```python
from build123d import *

# Parameters (mm, degrees)
SKETCH1_W                = 35.980750028
SKETCH1_H                = 26
BOSS_EXTRUDE1_DEPTH      = 2
LPATTERN1_COUNT          = 2
LPATTERN1_PITCH          = 4
BOSS_EXTRUDE2_DEPTH      = 6
BOSS_EXTRUDE2_DEPTH_BACK = 12
SKETCH2_W                = 35.980750028
SKETCH2_H                = 2
FILLET1_R                = 2
FILLET2_R                = 10
SKETCH4_R                = 5
CUT_EXTRUDE1_DEPTH       = 6


with BuildPart() as part:
    # Sketch1 → Boss-Extrude1 (new body)
    with BuildSketch(Plane.XY):
        with Locations((17.990375014, 13)):
            Rectangle(SKETCH1_W, SKETCH1_H)
    extrude(amount=BOSS_EXTRUDE1_DEPTH)


with BuildPart() as lpattern1_1:
    # LPattern1: pattern copy
    add(part.part.moved(Location(Vector(0, 0, 1) * (1 * LPATTERN1_PITCH))))


with BuildPart() as part_1:
    add(part.part)

    add(lpattern1_1.part)  # Boss-Extrude2 merges LPattern1_1
    # Sketch2 → Boss-Extrude2 (add, two sides: drawn at the far end of the back side and taken through both)
    with BuildSketch(Plane(origin=(0, 0, 0), x_dir=(-1, 0, 0), z_dir=(0, 0, -1)).offset(-BOSS_EXTRUDE2_DEPTH_BACK)):
        with Locations((-17.990375014, 1)):
            Rectangle(SKETCH2_W, SKETCH2_H)
    extrude(amount=BOSS_EXTRUDE2_DEPTH + BOSS_EXTRUDE2_DEPTH_BACK)

    # Fillet1
    fillet1_edges = [part_1.edges().sort_by_distance(p)[0] for p in [
        (17.990375014, 2, 0),
        (17.990375014, 2, 6),
    ]]
    fillet(fillet1_edges, radius=FILLET1_R)

    # Fillet2
    fillet2_edges = [part_1.edges().sort_by_distance(p)[0] for p in [
        (0, 26, 5),
        (35.980750028, 26, 5),
        (0, 26, 1),
        (35.980750028, 26, 1),
    ]]
    fillet(fillet2_edges, radius=FILLET2_R)

    # Sketch4 → Cut-Extrude1 (cut)
    with BuildSketch(Plane.XY.offset(6)):
        with Locations((17.990375014, 16.77)):
            Circle(SKETCH4_R)
    extrude(amount=-CUT_EXTRUDE1_DEPTH, mode=Mode.SUBTRACT)


solid = part_1.part
```
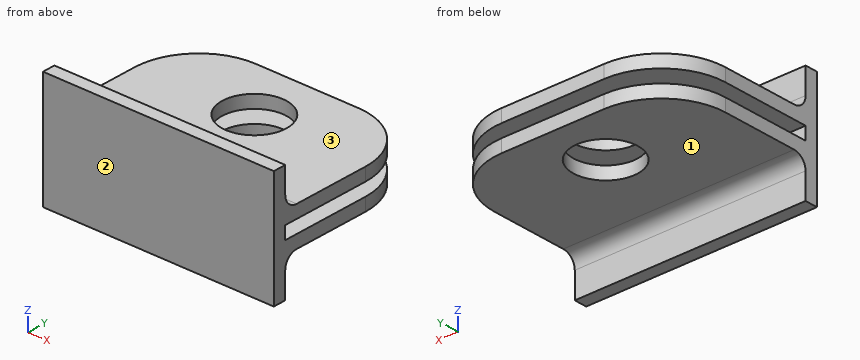
Verification items for the finished model (mm, model axes). Face numbers are marked on the shaded views. A direction names the side the tool comes from. Round coordinates to 2 decimals unless told otherwise and drop trailing zeros. Write each loop counter-clockwise with the first axis right and the second up, starting at its lowest first coordinate (ties: lowest second). Pieces come first, ordered by that corner, then holes. Notation, with made-up numbers: (11.25, 68.25) -> (56.25, 68.25) arc R26 ccw to (56.25, 95.25) -> close; hole circle Ø5 at (52.5, 24). An arc over 180 degrees is marked (long way). Write each question's results on one line, items separated by ' | '. Start each with the question number.
1. Set-up check for the marked faces 1, 2 and 3: record each of +Z, -Z, +X, -X, +Y, -Y from which the full face is reachable in a straight line by a thin tool's end or side.
2. Cross-section at B-B (x = 18). Enter the section's corners in (y, z).
3. Cross-section at D-D (x = 24.5). Enter the section's corners in (y, z).
4. Material ranges on probe 1 along Z at (x, y) = (23, 20.25); probe 2 along Y at (x, z) = (2, 3.75); probe 3 along Y at (x, z) = (22.5, 0.5), recorded low to high. Write a range as from..to.
5. Cross-section at A-A (y = 6.5). Enter the section's corners in (x, z).
6. Cross-section at C-C (y = 16.77). Enter the section's corners in (x, z).
7. Depth check by flat-ended pin: P1, Ø4.5, axis at x = 22, z = -5, coming from the +Y side; P2, Ø2, axis at x = 23.5, y = 5, coming from the -Z side; P3, Ø12, axis at x = 15.5, y = 9, coming from the +Z side; P4, Ø3, axis at x = 22.5, z = 8.5, coming from the -Y side. Enter the tip coordinate at first touch or a pass-through.
Solutions:
1) face 1: -Z, +X, -X, +Y | face 2: +Z, -Z, +X, -X, -Y | face 3: +Z, +X, -X, +Y
2) outline: (0, -6) -> (2, -6) -> (2, -2) arc R2 cw to (4, 0) -> (11.77, 0) -> (11.77, 2) -> (2, 2) -> (2, 4) -> (11.77, 4) -> (11.77, 6) -> (4, 6) arc R2 cw to (2, 8) -> (2, 12) -> (0, 12) -> close; (21.77, 0) -> (26, 0) -> (26, 2) -> (21.77, 2) -> close; (21.77, 4) -> (26, 4) -> (26, 6) -> (21.77, 6) -> close
3) outline: (0, -6) -> (2, -6) -> (2, -2) arc R2 cw to (4, 0) -> (26, 0) -> (26, 2) -> (2, 2) -> (2, 4) -> (26, 4) -> (26, 6) -> (4, 6) arc R2 cw to (2, 8) -> (2, 12) -> (0, 12) -> close
4) probe 1: z = 0..2, 4..6 | probe 2: y = 0..2 | probe 3: y = 0..14.61, 18.93..26
5) outline: (0, 0) -> (35.98, 0) -> (35.98, 2) -> (0, 2) -> close; (0, 4) -> (35.98, 4) -> (35.98, 6) -> (0, 6) -> close
6) outline: (0.03, 0) -> (12.99, 0) -> (12.99, 2) -> (0.03, 2) -> close; (0.03, 4) -> (12.99, 4) -> (12.99, 6) -> (0.03, 6) -> close; (22.99, 0) -> (35.95, 0) -> (35.95, 2) -> (22.99, 2) -> close; (22.99, 4) -> (35.95, 4) -> (35.95, 6) -> (22.99, 6) -> close
7) P1: stops at y = 2 | P2: stops at z = 0 | P3: stops at z = 6.27 | P4: stops at y = 0
